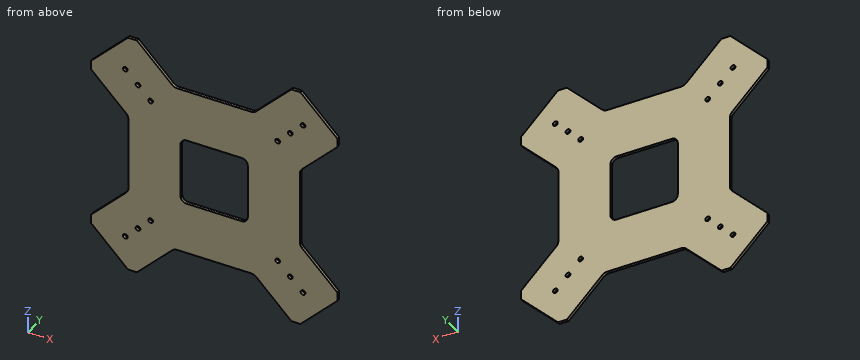
```python
from build123d import *

# Parameters (mm, degrees)
BOSS_EXTRUDE1_DEPTH  = 2
SKETCH2_W            = 45
SKETCH2_H            = 45
CUT_EXTRUDE1_DEPTH   = 117.689759619
FILLET1_R            = 4
CUT_EXTRUDE2_DEPTH   = 117.689759619
FILLET2_R            = 5
M3_CLEARANCE_HOLE1_D = 3.2


with BuildPart() as part:
    # Sketch1 → Boss-Extrude1 (new body)
    with BuildSketch(Plane(origin=(0, 0, 0), x_dir=(1, 0, 0), z_dir=(0, 1, 0))):
        Polygon((-57.751262658, 82.5), (-82.5, 57.751262658), (-82.5, -57.751262658), (-57.751262658, -82.5), (57.751262658, -82.5), (82.5, -57.751262658), (82.5, 57.751262658), (57.751262658, 82.5), align=None)
    extrude(amount=BOSS_EXTRUDE1_DEPTH)

    # Sketch2 → Cut-Extrude1 (cut, through all)
    with BuildSketch(Plane(origin=(0, 2, 0), x_dir=(1, 0, 0), z_dir=(0, 1, 0))):
        Rectangle(SKETCH2_W, SKETCH2_H)
    extrude(amount=-CUT_EXTRUDE1_DEPTH, mode=Mode.SUBTRACT)

    # Fillet1
    fillet1_edges = [part.edges().sort_by_distance(p)[0] for p in [
        (22.5, 1, -22.5),
        (22.5, 1, 22.5),
        (-22.5, 1, 22.5),
        (-22.5, 1, -22.5),
    ]]
    fillet(fillet1_edges, radius=FILLET1_R)

    # Sketch3 → Cut-Extrude2 (cut, through all)
    with BuildSketch(Plane(origin=(0, 2, 0), x_dir=(1, 0, 0), z_dir=(0, 1, 0))):
        Polygon((57.5, -26.751262658), (82.5, -51.751262658), (82.5, 51.751262658), (57.5, 26.751262658), align=None)
        Polygon((-51.751262658, -82.5), (51.751262658, -82.5), (26.751262658, -57.5), (-26.751262658, -57.5), align=None)
        Polygon((-57.5, 26.751262658), (-82.5, 51.751262658), (-82.5, -51.751262658), (-57.5, -26.751262658), align=None)
        Polygon((26.751262658, 57.5), (51.751262658, 82.5), (-51.751262658, 82.5), (-26.751262658, 57.5), align=None)
    extrude(amount=-CUT_EXTRUDE2_DEPTH, mode=Mode.SUBTRACT)

    # Fillet2
    fillet2_edges = [part.edges().sort_by_distance(p)[0] for p in [
        (-26.751262658, 1, -57.5),
        (26.751262658, 1, -57.5),
        (57.5, 1, 26.751262658),
        (57.5, 1, -26.751262658),
        (-26.751262658, 1, 57.5),
        (26.751262658, 1, 57.5),
        (-57.5, 1, -26.751262658),
        (-57.5, 1, 26.751262658),
    ]]
    fillet(fillet2_edges, radius=FILLET2_R)

    # M3 Clearance Hole1 (through all)
    with Locations(Plane(origin=(0, 0, 0), x_dir=(-1, 0, 0), z_dir=(0, -1, 0))):
        with Locations((-59.519029611, 59.519029611), (59.519029611, -59.519029611), (51.033748237, -51.033748237), (42.548466863, -42.548466863), (-59.519029611, -59.519029611), (-51.033748237, -51.033748237), (-42.548466863, -42.548466863), (59.519029611, 59.519029611), (51.033748237, 51.033748237), (42.548466863, 42.548466863), (-42.548466863, 42.548466863), (-51.033748237, 51.033748237)):
            Hole(M3_CLEARANCE_HOLE1_D / 2)


solid = part.part
```
The listing builds one solid part. Answer for the finished solid, in the listing's coordinates (mm). Coordinates: 2 decimals unless noted, no trailing zeros. Loops run counter-clockwise (first coordinate to the right, second up) from the corner with the lowest first, then second, coordinate; pieces in that order, holes last. Notation, with made-up numbers: M -10.5,64.5 L 31.5,64.5 A9 cw 31.5,75.5 Z; hole C -12,-10 d1. An arc over 180 degrees is marked long. Answer as a JSON object with one key per item and string values. Group by question number.
Item 1: Section A-A (z = -1) is taken. Write down the section's boundary in (x, y), and give its area (3 significant figures).
Item 2: Section C-C (x = -36.5) is taken. Write down the section's boundary in (y, z), and give its area (3 significant figures).
Item 3: Section B-B (x = 13.5) is taken. Write down the section's boundary in (y, z).
Item 4: Each of these flat-tipped pins is pushed along its axis until it touches: P1, Ø1, axis at x = -5.5, y = 1, coming from the -Z side; P2, Ø1, axis at y = 0.5, z = -50.5, coming from the +X side; P3, Ø1, axis at y = 1, z = -7.5, coming from the -X side. Where does it stop, or does it pass through?
Item 5: Section D-D (y = 1.4) is taken. Give the number of separate pieces and of enclosed holes in the cut face, and give its area (3 significant figures).
Item 6: Consider L1, parallel to Z at x = -3, y = 1.2; L2, parallel to Z at x = 59.5, y = 1.55. Determine where each line is inside the solid, lowest interval first.
Solved:
{
 "1": {"outline": "M -57.5,0 L -22.5,0 L -22.5,2 L -57.5,2 Z; M 22.5,0 L 57.5,0 L 57.5,2 L 22.5,2 Z", "area": "140 mm2"},
 "2": {"outline": "M 0,-67.25 L 2,-67.25 L 2,67.25 L 0,67.25 Z", "area": "269 mm2"},
 "3": {"outline": "M 0,-57.5 L 2,-57.5 L 2,-22.5 L 0,-22.5 Z; M 0,22.5 L 2,22.5 L 2,57.5 L 0,57.5 Z"},
 "4": {"P1": "stops at z = -57.5", "P2": "stops at x = 81.75", "P3": "stops at x = -57.5"},
 "5": {"separate pieces": "1", "enclosed holes": "13", "area": "16,000 mm2"},
 "6": {"L1": "z = -57.5 to -22.5, 22.5 to 57.5", "L2": "z = -80.75 to -61.12, -57.92 to -28.75, 28.75 to 57.92, 61.12 to 80.75"}
}
